Design review of the part built by this model. Coordinates are the model's own, in mm. A direction names the side the tool comes from. Coordinates: 2 decimals unless noted, no trailing zeros. Order: outer loops, then holes, each group sorted by start corner. A loop starts at its lowest first (then second) coordinate and runs counter-clockwise, first axis right, second up. Notation, with made-up numbers: (35, -23.75) -> (53, -23.75) arc R15 ccw to (53, 2.25) -> close; hole circle Ø3 at (59, 36.5). An arc over 180 degrees is marked (long way). Use a Markdown table: item, result. Add a question column.
Q1. Add section B-B (z = 0). State the section outline as (x, y) points, then the cut area to 3 significant figures.
Q2. Add section A-A (y = 195). State the section outline as (x, z) points, then the cut area to 3 significant figures.
Q3. Add section D-D (z = 274.5). State the section outline as (x, y) points, then the cut area to 3 significant figures.
Q4. Machinability: for faces 4 (the face through (12.932, 83.373, 5.362)), 5 (the face through (-1.73, 217.4, 7.81)), 6 (the face through (0, 225, 0)), 7 (the face through (5.1, 165, -9.4)), 8 (the face through (-0.976, 202.436, 193.229)), which of the approach directions +Z, -Z, +X, -X, +Y, -Y give a long, thin tool a straight path to every point of the face, cutting with its end or side? Answer none if there is none.
Q5. The part is to be moulded in two halves that separate along Y. For faces 1 (the face through (-0.976, 202.436, -35.469)), 2 (the face through (0, 195, -50)), 3 (the face through (10, 172.4, -3.2)), say which applies: pulls with the +Y half, pulls with the -Y half, needs draft (parallel to the pull), parting line crosses it, or undercut.
Q6. Wall thickness on probe 1 along Y at (x, z) = (14, -11); probe 2 along Y at (x, z) = (18.5, 14); probe 3 along Z at (x, y) = (-3.5, 134): over which ranges is each line inside the solid? List them lowest first.
Q7. Insertion check: pin 1 (8 mm diameter, centred on y = 180, z = 294.5, fed in from -X); pin 2 (5 mm diameter, centred on x = -8.5, z = 41, fed in from +Y); pin 3 (10 mm diameter, centred on x = -16, y = 142, fed in from +Z); pin 4 (3 mm diameter, centred on x = 8, z = 287, fed in from -Y). Each pin has a flat end and moves straight along its axis. Give the tip position at first contact, or say it passes through.
from build123d import *

# Parameters (mm, degrees)
SKETCH_1_R           = 14
EXTRUDE_1_DEPTH      = 165
SKETCH_2_R           = 10.5
EXTRUDE_2_DEPTH      = 15
CHAMFER_2_SIZE       = 4
SKETCH_4_R           = 24
EXTRUDE_3_DEPTH      = 30
SKETCH_5_R           = 8
EXTRUDE_4_DEPTH      = 15
SKETCH_6_R           = 7.5
EXTRUDE_5_DEPTH      = 370
EXTRUDE_5_DEPTH_BACK = 50
CHAMFER_3_SIZE       = 1.5


with BuildPart() as part:
    # 草图1 → 凸台-拉伸1 (new body)
    with BuildSketch(Plane(origin=(0, 0, 0), x_dir=(1, 0, 0), z_dir=(0, 1, 0))):
        Circle(SKETCH_1_R)
    extrude(amount=EXTRUDE_1_DEPTH)

    # 草图2 → 凸台-拉伸2 (add)
    with BuildSketch(Plane(origin=(0, 165, 0), x_dir=(1, 0, 0), z_dir=(0, 1, 0))):
        Circle(SKETCH_2_R)
    extrude(amount=EXTRUDE_2_DEPTH)

    # 倒角2
    chamfer_2_edges = [part.edges().sort_by_distance(p)[0] for p in [
        (-14, 0, 0),
    ]]
    chamfer(chamfer_2_edges, length=CHAMFER_2_SIZE)

    # 草图4 → 凸台-拉伸3 (add)
    with BuildSketch(Plane(origin=(0, 180, 0), x_dir=(1, 0, 0), z_dir=(0, 1, 0))):
        Circle(SKETCH_4_R)
    extrude(amount=EXTRUDE_3_DEPTH)

    # 草图5 → 凸台-拉伸4 (add)
    with BuildSketch(Plane(origin=(0, 210, 0), x_dir=(1, 0, 0), z_dir=(0, 1, 0))):
        Circle(SKETCH_5_R)
    extrude(amount=EXTRUDE_4_DEPTH)

    # 草图6 → 凸台-拉伸5 (add, two sides)
    with BuildSketch(Plane.XY) as extrude_5_sk:
        with Locations((0, 195)):
            Circle(SKETCH_6_R)
    extrude(amount=EXTRUDE_5_DEPTH)
    extrude(extrude_5_sk.sketch, amount=-EXTRUDE_5_DEPTH_BACK)

    # 倒角3
    chamfer_3_edges = [part.edges().sort_by_distance(p)[0] for p in [
        (-24, 180, 0),
        (-24, 210, 0),
        (-7.5, 195, -50),
        (-7.5, 195, 370),
    ]]
    chamfer(chamfer_3_edges, length=CHAMFER_3_SIZE)


solid = part.part
Established:
| question | item | result |
|---|---|---|
| 1 | outline | (-24, 181.5) -> (-22.5, 180) -> (-10.5, 180) -> (-10.5, 165) -> (-14, 165) -> (-14, 4) -> (-10, 0) -> (10, 0) -> (14, 4) -> (14, 165) -> (10.5, 165) -> (10.5, 180) -> (22.5, 180) -> (24, 181.5) -> (24, 208.5) -> (22.5, 210) -> (8, 210) -> (8, 225) -> (-8, 225) -> (-8, 210) -> (-22.5, 210) -> (-24, 208.5) -> close |
| 1 | area | 6,590 mm^2 |
| 2 | outline | (-7.5, -48.5) -> (-6, -50) -> (6, -50) -> (7.5, -48.5) -> (7.5, -22.8) arc R24 ccw to (7.5, 22.8) -> (7.5, 368.5) -> (6, 370) -> (-6, 370) -> (-7.5, 368.5) -> (-7.5, 22.8) arc R24 ccw to (-7.5, -22.8) -> close |
| 2 | area | 7,400 mm^2 |
| 3 | outline | circle Ø15 at (0, 195) |
| 3 | area | 177 mm^2 |
| 4 | face 4 | -Y |
| 4 | face 5 | +Y |
| 4 | face 6 | +Z, -Z, +X, -X, +Y |
| 4 | face 7 | none |
| 4 | face 8 | +Z |
| 5 | face 1 | parting line crosses it |
| 5 | face 2 | needs draft |
| 5 | face 3 | undercut |
| 6 | probe 1 | 180 to 210 |
| 6 | probe 2 | 180.7 to 209.3 |
| 6 | probe 3 | -13.56 to 13.56 |
| 7 | pin 1 | through |
| 7 | pin 2 | y = 199.5 |
| 7 | pin 3 | z = 8.66 |
| 7 | pin 4 | y = 191.26 |
